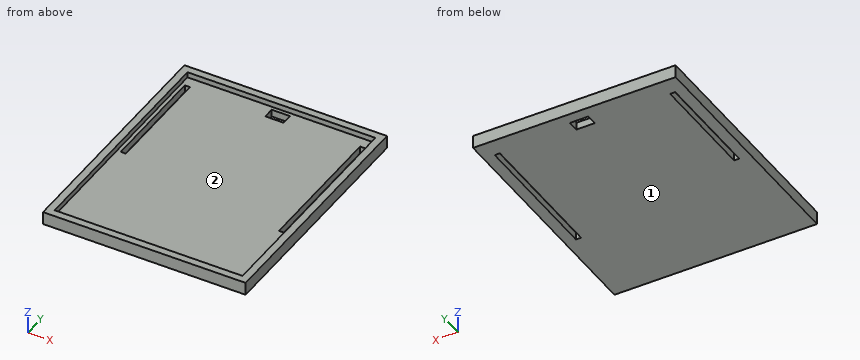
```python
from build123d import *

# Parameters (mm, degrees)
F0_W     = 69.85
F0_H     = 4.445
F1_DEPTH = 42.037
F2_T     = -2.54
F3_W     = 1.778
F3_H     = 38.1
F3_W_2   = 6.35
F3_H_2   = 3.81
F3_H_3   = 48.26
F4_DEPTH = 25.4


with BuildPart() as f1:
    # F0 (on Front) → F1 (new body, symmetric)
    with BuildSketch(Plane.XZ):
        with Locations((2.62026, -14.102518)):
            Rectangle(F0_W, F0_H)
    extrude(amount=F1_DEPTH, both=True)

    # F2
    f2_openings = [f1.faces().sort_by_distance(p)[0] for p in [
        (2.62026, 0, -11.880018),
    ]]
    offset(amount=F2_T, openings=f2_openings)

    # F3 (on face) → F4 (cut)
    with BuildSketch(Plane(origin=(0, 0, -16.325018), x_dir=(1, 0, 0), z_dir=(0, 0, -1))):
        with Locations((-27.60574, -16.637)):
            Rectangle(F3_W, F3_H)
        with Locations((3.175, -36.322)):
            Rectangle(F3_W_2, F3_H_2)
        with Locations((32.84626, -11.557)):
            Rectangle(F3_W, F3_H_3)
    extrude(amount=-F4_DEPTH, mode=Mode.SUBTRACT)


solid = f1.part
```
Input: part model. Units: mm. Frame: model coordinates. Face numbers are marked on the shaded views. Coordinates: 2 decimals unless noted, no trailing zeros. Loops run counter-clockwise (first coordinate to the right, second up) from the corner with the lowest first, then second, coordinate; pieces in that order, holes last. Notation, with made-up numbers: M 59,50.5 L 73,50.5 A29 ccw 73,77.5 Z; hole C 4.5,-12.75 d10. An arc over 180 degrees is marked long. One line per item, written item: value.
(1) Section D-D (z = -14.9). Output: boundary loops of the cut face in (x, y).
Filled in:
outline: M -32.3,-42.04 L 37.55,-42.04 L 37.55,42.04 L -32.3,42.04 Z; hole M -28.49,-2.41 L -26.72,-2.41 L -26.72,35.69 L -28.49,35.69 Z; hole M 0,34.42 L 6.35,34.42 L 6.35,38.23 L 0,38.23 Z; hole M 31.96,-12.57 L 33.74,-12.57 L 33.74,35.69 L 31.96,35.69 Z
(2) Line query: line 1 along X through (y, z) = (21, -15.1); line 2 along X through (y, z) = (35, -14.9); line 3 along X through (y, z) = (1.5, -13.55). Output: solid intervals per line, ascending. Write a range as from..to.
Filled in:
line 1: -32.3..-28.49, -26.72..31.96, 33.74..37.55
line 2: -32.3..-28.49, -26.72..0, 6.35..31.96, 33.74..37.55
line 3: -32.3..-29.76, 35.01..37.55
(3) Pull-direction query (Y, two-part tool) for the marked faces 1 and 2; classes: +Y half, -Y half, draft (parallel to the pull), parting line (faces both ways), or undercut.
Filled in:
face 1: draft
face 2: undercut
(4) Section A-A (x = 2.5). Output: boundary loops of the cut face in (y, z), and give its area (3 significant figures).
Filled in:
outline: M -42.04,-16.33 L 34.42,-16.33 L 34.42,-13.79 L -39.5,-13.79 L -39.5,-11.88 L -42.04,-11.88 Z; M 38.23,-16.33 L 42.04,-16.33 L 42.04,-11.88 L 39.5,-11.88 L 39.5,-13.79 L 38.23,-13.79 Z
area: 214 mm^2
(5) Section B-B (y = -5). Output: boundary loops of the cut face in (x, z).
Filled in:
outline: M -32.3,-16.33 L 31.96,-16.33 L 31.96,-13.79 L -29.76,-13.79 L -29.76,-11.88 L -32.3,-11.88 Z; M 33.74,-16.33 L 37.55,-16.33 L 37.55,-11.88 L 35.01,-11.88 L 35.01,-13.79 L 33.74,-13.79 Z
(6) Section C-C (y = 13). Output: boundary loops of the cut face in (x, z).
Filled in:
outline: M -32.3,-16.33 L -28.49,-16.33 L -28.49,-13.79 L -29.76,-13.79 L -29.76,-11.88 L -32.3,-11.88 Z; M -26.72,-16.33 L 31.96,-16.33 L 31.96,-13.79 L -26.72,-13.79 Z; M 33.74,-16.33 L 37.55,-16.33 L 37.55,-11.88 L 35.01,-11.88 L 35.01,-13.79 L 33.74,-13.79 Z
(7) Pin query (flat end, axial travel): pin 1 (1 mm diameter, centred on x = 27, y = -29.5, fed in from +Z) (3 decimals). Return the tip coordinate at first contact, or that it passes through.
Filled in:
pin 1: z = -13.785
